Input: part model. Units: mm. Frame: model coordinates. Face numbers are marked on the shaded views. A direction names the side the tool comes from. Round coordinates to 2 decimals unless told otherwise and drop trailing zeros. Order: outer loops, then holes, each group sorted by start corner. A loop starts at its lowest first (then second) coordinate and runs counter-clockwise, first axis right, second up. Notation, with made-up numbers: M -5,48 L 33,48 A19 ccw 33,72 Z; hole C -37,-33 d4. An arc over 180 degrees is marked long. One line per question, with ' | ' between items.
Autodesk Inventor part; units mm, degrees
ref_plane "YZ Plane" through (0, 0, 0) normal (1, 0, 0) x (0, 1, 0)
ref_plane "XZ Plane" through (0, 0, 0) normal (0, 1, 0) x (-1, 0, 0)
ref_plane "XY Plane" through (0, 0, 0) normal (0, 0, 1) x (1, 0, 0)
sketch "Szkic1" plane through (0, 0, 0) normal (0, 0, 1) x (1, 0, 0)
  line L0 (-10.1243, 0) -> (60.0207, 0)
  line L1 (0, -10.1243) -> (0, 60.0207)
  line L2 (0, 50) -> (0, 0.5)
  line L3 (0.5, 0) -> (50, 0)
  line L4 (50, 2) -> (2.5, 2)
  line L5 (2, 2.5) -> (2, 50)
  line L6 (2, 50) -> (0, 50)
  line L7 (50, 0) -> (50, 2)
  arc A0 (2, 2.5) -> (2.5, 2) centre (2.5, 2.5) ccw
  arc A1 (0, 0.5) -> (0.5, 0) centre (0.5, 0.5) ccw
  point P0 (0, 0)
  dimension "d0" = 2
  dimension "d2" = 2
  dimension "d3" = 50
  dimension "d4" = 50
  dimension "d5" = 0.5
extrude "Wyciągnięcie proste1" add sketch "Szkic1" along normal blind 300 contours A1 L1 L6 L5 A0 L4 L7 L0
sketch "Szkic2" plane through (2.5, 2, 0) normal (0, 1, 0) x (1, 0, 0)
  line L0 (-2.5, 0) -> (-2.5, -300)
  line L1 (0, 0) -> (-0.5, 0)
  line L2 (-0.5, 0) -> (-0.5, -300)
  line L3 (0, -300) -> (-0.5, -300)
  line L4 (0, 0) -> (0, -300)
  line L5 (47.5, -300) -> (-0.5, -300)
  line L6 (-0.5, -300) -> (-0.5, -252)
  line L7 (-0.5, -252) -> (47.5, -252)
  line L8 (47.5, -252) -> (47.5, -300)
  line L9 (47.5, 0) -> (-0.5, 0)
  line L10 (-0.5, 0) -> (-0.5, -48)
  line L11 (-0.5, -48) -> (47.5, -48)
  line L12 (47.5, -48) -> (47.5, 0)
  dimension "d8" = 48
  dimension "d9" = 48
extrude "Wyciągnięcie proste2" cut sketch "Szkic2" against normal through all contours L4 L11 L2 L1 | L9 L12 L11 L4 | L7 L8 L5 L4 | L4 L3 L2 L7
sketch "Szkic3" plane through (2, 2.5, 0) normal (1, 0, 0) x (0, 0, -1)
  line L0 (0, 0) -> (0, 47.5)
  line L1 (0, 47.5) -> (-300, 47.5)
  circle A0 centre (-20, 17.5) radius 3.5
  point P0 (0, -2.5)
  dimension "d12" = 20
  dimension "d13" = 30
  dimension "d14" = 7
extrude "Wyciągnięcie proste3" cut sketch "Szkic3" against normal through all
pattern_linear "Szyk prostokątny1" count 2 spacing 15 along (0, 0, 1) of "Wyciągnięcie proste3"
sketch "Szkic4" plane through (2, 2.5, 0) normal (1, 0, 0) x (0, 0, -1)
  line L0 (0, 47.5) -> (-300, 47.5)
  line L1 (0, 0) -> (-300, 0)
  line L2 (-160, 15) -> (-140, 15)
  line L3 (-140, 15) -> (-140, 5)
  line L4 (-140, 5) -> (-160, 5)
  line L5 (-160, 5) -> (-160, 15)
  line L6 (-150, 47.5) -> (-150, -7.9092) construction
  line L7 (-48, -0.5) -> (-252, -0.5)
  point P0 (0, -2.5)
  dimension "d20" = 20
  dimension "d21" = 10
  dimension "d22" = 5
extrude "Wyciągnięcie proste4" cut sketch "Szkic4" against normal through all
properties part number "kątownik 3" material "Aluminium 6061"
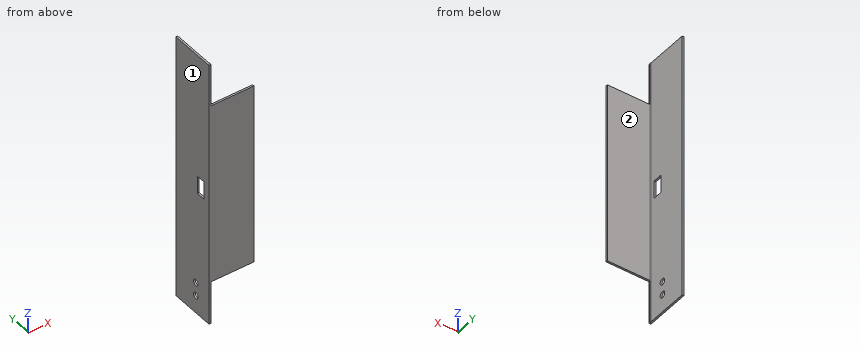
Item 1: Section query A-A, the plane z = 20. Return loops of the section in (x, y).
Report:
outline: M 0,0.5 A0.5 ccw 0.5,0 L 2,0 L 2,2 L 2.5,2 A0.5 cw 2,2.5 L 2,16.5 L 0,16.5 Z; M 0,23.5 L 2,23.5 L 2,50 L 0,50 Z
Item 2: Access query for the marked faces 1 and 2. Directions: +Z, -Z, +X, -X, +Y, -Y. A direction counts if a zero-diameter tool reaches every point of the face in a straight line with its end or side. Return the directions, or none.
Report:
face 1: +Z, -Z, -X, +Y, -Y | face 2: +Z, -Z, +X, +Y
Item 3: Section query C-C, the plane z = 64.5. Return loops of the section in (x, y), plus the area to 3 significant figures.
Report:
outline: M 0,0.5 A0.5 ccw 0.5,0 L 50,0 L 50,2 L 2.5,2 A0.5 cw 2,2.5 L 2,50 L 0,50 Z | area: 196 mm²
Item 4: Section query D-D, the plane x = 9. Return loops of the section in (y, z).
Report:
outline: M 0,48 L 2,48 L 2,252 L 0,252 Z
Item 5: Section query B-B, the plane y = 11. Return loops of the section in (x, z).
Report:
outline: M 0,0 L 2,0 L 2,140 L 0,140 Z; M 0,160 L 2,160 L 2,300 L 0,300 Z
Item 6: Line query: line 1 along Y through (x, z) = (0.9, 35); line 2 along X through (y, z) = (27.5, 132). Output: solid intervals per line, ascending. Write a range as from..to.
Report:
line 1: 0..16.5, 23.5..50 | line 2: 0..2
Item 7: First-contact query: pin 1 (4 mm diameter, centred on x = 42.5, z = 211.5, fed in from +Y); pin 2 (1 mm diameter, centred on y = 1, z = 17.5, fed in from +X); pin 3 (5 mm diameter, centred on x = 6.5, y = 6, fed in from -Z); pin 4 (1.6 mm diameter, centred on x = 0.5, z = 147, fed in from -Y). Flat tips, straight axial feed; report the tip coordinate or a pass-through.
Report:
pin 1: y = 2 | pin 2: x = 2 | pin 3: through | pin 4: y = 0
